The listing builds one solid part. Answer for the finished solid, in the listing's coordinates (mm). Face numbers are marked on the shaded views. A direction names the side the tool comes from. Give positions to 0.01 mm unless a question says otherwise; leave off trailing zeros. Write each loop counter-clockwise with the first axis right and the second up, starting at its lowest first coordinate (ties: lowest second). Pieces come first, ordered by that corner, then holes. Notation, with made-up numbers: (74, -22.5) - (110, -22.5) arc R13 ccw to (110, 2.5) - close; hole circle Ø10 at (52.25, 52.5). An arc over 180 degrees is marked (long way). Return JSON: item names as keys, results as strings.
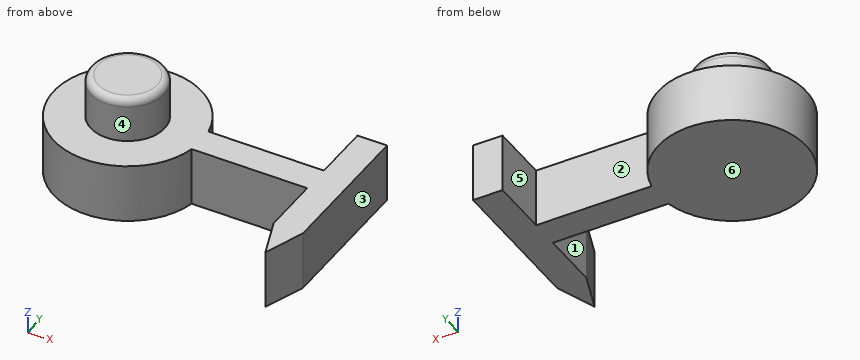
Autodesk Inventor part; units mm, degrees
ref_plane "YZ Plane" through (0, 0, 0) normal (1, 0, 0) x (0, 1, 0)
ref_plane "XZ Plane" through (0, 0, 0) normal (0, 1, 0) x (-1, 0, 0)
ref_plane "XY Plane" through (0, 0, 0) normal (0, 0, 1) x (1, 0, 0)
sketch "Esboço1" plane through (0, 0, 0) normal (0, 0, 1) x (1, 0, 0)
  arc A0 (4.899, 1) -> (4.899, -1) centre (0, 0) ccw
  line L0 (14.72, 0) -> (14.72, 1)
  line L1 (12.72, 1) -> (4.899, 1)
  line L2 (0, 0) -> (14.72, 0) construction
  line L3 (14.72, 0) -> (14.72, -1)
  line L4 (12.7254, -1) -> (4.899, -1)
  line L5 (12.72, 5) -> (14.72, 5)
  line L6 (14.72, 5) -> (14.72, -5)
  line L7 (14.72, -5) -> (12.7254, -5) construction
  line L8 (12.7254, -5) -> (12.7254, -1)
  line L9 (12.72, 1) -> (12.72, 5)
  line L10 (12.7254, -5) -> (13.7254, -7.74)
  line L11 (14.72, -5) -> (13.7254, -7.74)
  dimension "d9" = 10
  dimension "d10" = 1
  dimension "d11" = 1
  dimension "d13" = 2
  dimension "d14" = 10
  dimension "d15" = 4
  dimension "d16" = 4
  dimension "d18" = 40
  dimension "d19" = 2.74
extrude "Extrusão1" add sketch "Esboço1" along normal mid plane 4
sketch "Esboço2" plane through (0, 0, 2) normal (0, 0, 1) x (1, 0, 0)
  circle A0 centre (0, 0) radius 2.5
  dimension "d22" = 5
extrude "Extrusão2" add sketch "Esboço2" along normal blind 3
fillet "Arredondamento1" radius 0.5 1 edges at (-2.5, 0, 5)
properties part number "solda"
Item 1: Consider L1, parallel to Y at x = 10.5, z = 1.75; L2, parallel to Z at x = 4.5, y = 0.25; L3, parallel to X at y = -1.75, z = -1.5. Determine where each line is inside the solid, lowest interval first.
Answer below:
{"L1": "y = -1 to 1", "L2": "z = -2 to 2", "L3": "x = -4.68 to 4.68, 12.73 to 14.72"}
Item 2: A cutting plane is placed at C-C on y = 0. Determine the outline of the cut face in (x, z), then the cut area to 3 significant figures.
Answer below:
{"outline": "(-5, -2) - (14.72, -2) - (14.72, 2) - (2.5, 2) - (2.5, 4.5) arc R0.5 ccw to (2, 5) - (-2, 5) arc R0.5 ccw to (-2.5, 4.5) - (-2.5, 2) - (-5, 2) - close", "area": "93.8 mm²"}
Item 3: A cutting plane is placed at B-B on x = 0. Determine the outline of the cut face in (y, z).
Answer below:
{"outline": "(-5, -2) - (5, -2) - (5, 2) - (2.5, 2) - (2.5, 4.5) arc R0.5 ccw to (2, 5) - (-2, 5) arc R0.5 ccw to (-2.5, 4.5) - (-2.5, 2) - (-5, 2) - close"}
Item 4: Flat-ended cylindrical pins translate along their axes: P1, Ø2, axis at y = -3, z = -0.5, coming from the -X side; P2, Ø1.2, axis at x = 8.5, z = 0.5, coming from the +Y side; P3, Ø3, axis at x = 9.5, z = -1, coming from the -Y side. Find the tip coordinate at first contact, or state that the pin passes through.
Answer below:
{"P1": "stops at x = -4.58", "P2": "stops at y = 1", "P3": "stops at y = -1"}
Item 5: For the marked faces 1, 2 and 3, determine the directions among +Z, -Z, +X, -X, +Y, -Y from which every point of the face is accessible in a straight line to the end or side of a thin tool.
Answer below:
{"face 1": "+Z, -Z, -Y", "face 2": "+Z, -Z, +Y", "face 3": "+Z, -Z, +X, +Y, -Y"}
Item 6: A cutting plane is placed at A-A on z = -0.25. Determine the outline of the cut face in (x, y).
Answer below:
{"outline": "(4.9, -1) - (12.73, -1) - (12.73, -5) - (13.73, -7.74) - (14.72, -5) - (14.72, 5) - (12.72, 5) - (12.72, 1) - (4.9, 1) arc R5 ccw (long way) to start"}
Item 7: The mould has two halves that part along X. Classify the marked faces 4, 5 and 6: +X half, -X half, draft (parallel to the pull), parting line (faces both ways), or undercut.
Answer below:
{"face 4": "parting line", "face 5": "undercut", "face 6": "draft"}
Item 8: A cutting plane is placed at D-D on x = 9. Determine the outline of the cut face in (y, z), then the cut area to 3 significant figures.
Answer below:
{"outline": "(-1, -2) - (1, -2) - (1, 2) - (-1, 2) - close", "area": "8.00 mm²"}
